from build123d import *

# Parameters (mm, degrees)
ESTRUSIONE_ESTRUSIONE1_DEPTH = 2.8
SCHIZZO3_R                   = 1.625
TAGLIO_ESTRUSIONE1_DEPTH     = 3.8


with BuildPart() as part:
    # Schizzo1 → Estrusione-Estrusione1 (new body)
    with BuildSketch(Plane(origin=(0, 0, 0), x_dir=(1, 0, 0), z_dir=(0, 1, 0))):
        with BuildLine():
            Line((0, 12.183185174), (0, 9.95))
            ThreePointArc((0, 9.95), (7.035712473, 7.035712473), (9.95, 0))
            ThreePointArc((9.95, 0), (9.159023292, -3.887774728), (6.911850786, -7.157431013))
            ThreePointArc((6.911850786, -7.157431013), (6.843976854, -11.045925983), (10.732471824, -11.113799915))
            ThreePointArc((10.732471824, -11.113799915), (14.221799986, -6.036795935), (15.45, 0))
            ThreePointArc((15.45, 0), (10.924799769, 10.924799769), (0, 15.45))
            Line((0, 15.45), (0, 12.183185174))
        make_face()
        with BuildLine():
            ThreePointArc((0, 15.45), (-2.75, 12.7), (0, 9.95))
            Line((0, 9.95), (0, 12.183185174))
            Line((0, 12.183185174), (0, 15.45))
        make_face()
    extrude(amount=-ESTRUSIONE_ESTRUSIONE1_DEPTH)

    # Schizzo3 → Taglio-Estrusione1 (cut, through all)
    with BuildSketch(Plane(origin=(0, 0, 0), x_dir=(1, 0, 0), z_dir=(0, 1, 0))):
        with Locations((0, 12.7)):
            Circle(SCHIZZO3_R)
        with Locations((8.822161305, -9.135615464)):
            Circle(SCHIZZO3_R)
    extrude(amount=-TAGLIO_ESTRUSIONE1_DEPTH, mode=Mode.SUBTRACT)


solid = part.part
Input: part model. Units: mm. Frame: model coordinates. Coordinates: 2 decimals unless noted, no trailing zeros. Loops run counter-clockwise (first coordinate to the right, second up) from the corner with the lowest first, then second, coordinate; pieces in that order, holes last. Notation, with made-up numbers: (77.5, 51.5) -> (108.5, 51.5) arc R6 ccw to (108.5, 59.5) -> close; hole circle Ø11 at (52.25, 14.5). An arc over 180 degrees is marked (long way). Write each question's results on one line, items separated by ' | '. Start each with the question number.
Q1. Section A-A, the plane z = -12.7. Return the cut outline in (x, y) (3 decimals), plus the area to 3 significant figures.
Q2. Section B-B, the plane y = -2. Return the cut outline in (x, z) (3 decimals), plus the area to 3 significant figures.
Q3. Pull-direction query (Z, two-part tool) for faces 1 (the flat face through (10, 0, -5)), 2 (the cylindrical face through (-2.75, -1.38, -12.76)), 3 (the cylindrical face through (7.2, -1.38, 9.06)); classes: released by +Z, released by -Z, zero draft, split by the parting line, or undercut.
Q4. Section C-C, the plane x = 3.5. Return the cut outline in (y, z), plus the area to 3 significant figures.
Q5. Section D-D, the plane x = 11. Return the cut outline in (y, z), plus the area to 3 significant figures.
Q6. Ray query, line 1 (Z direction, x = 8.75, y = -2.05); line 2 (X direction, y = -1, z = 9); line 3 (X direction, y = -0.65, z = -12.7) (3 decimals). Return the intervals inside material, ascending. Write a range as from..to.
Q7. Pin query (flat end, axial travel): pin 1 (1.5 mm diameter, centred on y = -2, z = 7.5, fed in from +X); pin 2 (1.9 mm diameter, centred on x = 0, z = -12.7, fed in from -Y); pin 3 (1 mm diameter, centred on x = 2, y = -2.5, fed in from -Z). Return the tip coordinate at first contact, or that it passes through.
Found:
1) outline: (-2.75, -2.8) -> (-1.625, -2.8) -> (-1.625, 0) -> (-2.75, 0) -> close; (1.625, -2.8) -> (8.798, -2.8) -> (8.798, 0) -> (1.625, 0) -> close | area: 23.2 mm2
2) outline: (0, -15.45) arc R15.45 ccw to (10.732, 11.114) arc R2.75 ccw to (6.912, 7.157) arc R9.95 cw to (0, -9.95) arc R2.75 ccw to start; hole circle Ø3.25 at (0, -12.7); hole circle Ø3.25 at (8.822, 9.136) | area: 173 mm2
3) face 1: zero draft | face 2: split by the parting line | face 3: undercut
4) outline: (-2.8, -15.05) -> (0, -15.05) -> (0, -9.31) -> (-2.8, -9.31) -> close | area: 16.1 mm2
5) outline: (-2.8, -10.85) -> (0, -10.85) -> (0, 10.85) -> (-2.8, 10.85) -> close | area: 60.8 mm2
6) line 1: -12.73..-4.74, 4.74..7.51, 10.76..11.88 | line 2: 6.08..7.2, 10.44..12.56 | line 3: -2.75..-1.625, 1.625..8.798
7) pin 1: x = 13.9 | pin 2: through | pin 3: z = -15.38
